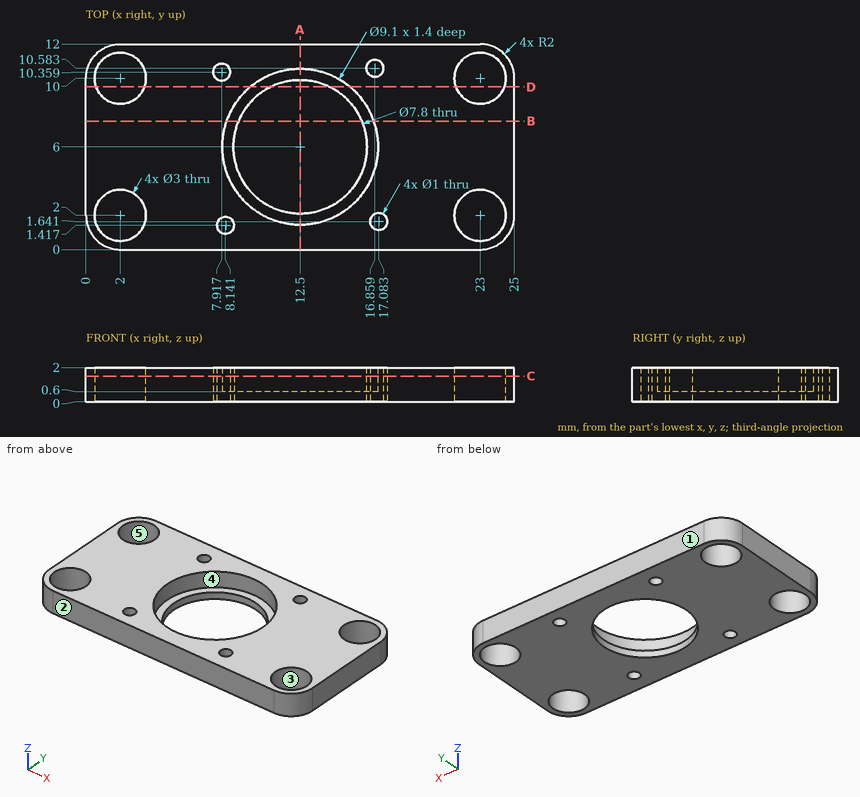
Here's the drawing with two shaded views (mm, measured from the low corner). I have some questions. A direction names the side the tool comes from. Coordinates: 2 decimals unless noted, no trailing zeros. Order: outer loops, then holes, each group sorted by start corner. A loop starts at its lowest first (then second) coordinate and runs counter-clockwise, first axis right, second up. Notation, with made-up numbers: (82, -26.75) - (140, -26.75) arc R26 cw to (140, 8.25) - close; hole circle Ø3 at (-8, 21). An arc over 180 degrees is marked (long way). Use CSV: the item, a comma, the result in double quotes. Start each with the question number.
1. Suppose I cut it at D-D on y = 9.5. List the corners of the cut face in (x, z) for me, then the cut area to 3 significant figures.
2. If we mould it in two halves opening along Y, with no side actions, what happens to the marked faces 1, 2 and 3? For each: +Y half, -Y half, draft (parallel to the pull), parting line (faces both ways), or undercut.
3. For the marked faces 4 and 5, which set-ups out of +Z, -Z, +X, -X, +Y, -Y let a thin tool reach every point of the face, with its end or its side?
4. Please list where these lines run through material, in increasing order: line 1 (Y direction, x = 2, z = 0.6); line 2 (X direction, y = 10, z = 1.05) (1 decimal); line 3 (X direction, y = 9.5, z = 1.45) (1 decimal). Write a range as from..to.
5. Suppose I cut it at B-B on y = 7.5. List the corners of the cut face in (x, z) for me.
6. Suppose I cut it at A-A on x = 12.5. List the corners of the cut face in (y, z) for me.
7. Suppose I cut it at C-C on z = 1.5. Give the number of separate pieces and of enclosed holes in the cut face, then the cut area to 3 significant figures.
Output:
1,outline,"(0, 0) - (0.59, 0) - (0.59, 2) - (0, 2) - close; (3.41, 0) - (10.78, 0) - (10.78, 0.6) - (9.59, 0.6) - (9.59, 2) - (3.41, 2) - close; (14.22, 0) - (21.59, 0) - (21.59, 2) - (15.41, 2) - (15.41, 0.6) - (14.22, 0.6) - close; (24.41, 0) - (25, 0) - (25, 2) - (24.41, 2) - close"
1,area,"28.5 mm2"
2,face 1,"+Y half"
2,face 2,"-Y half"
2,face 3,"undercut"
3,face 4,"+Z"
3,face 5,"+Z, -Z"
4,line 1,"y = 0..0.5, 3.5..8.5, 11.5..12"
4,line 2,"x = 0..0.5, 3.5..7.6, 8.3..10.3, 14.7..21.5, 24.5..25"
4,line 3,"x = 0..0.6, 3.4..9.6, 15.4..21.6, 24.4..25"
5,outline,"(0, 0) - (8.9, 0) - (8.9, 0.6) - (8.2, 0.6) - (8.2, 2) - (0, 2) - close; (16.1, 0) - (25, 0) - (25, 2) - (16.8, 2) - (16.8, 0.6) - (16.1, 0.6) - close"
6,outline,"(0, 0) - (2.1, 0) - (2.1, 0.6) - (1.45, 0.6) - (1.45, 2) - (0, 2) - close; (9.9, 0) - (12, 0) - (12, 2) - (10.55, 2) - (10.55, 0.6) - (9.9, 0.6) - close"
7,separate pieces,"1"
7,enclosed holes,"9"
7,area,"200 mm2"
